The listing builds one solid part. Answer for the finished solid, in the listing's coordinates (mm). Face numbers are marked on the shaded views. A direction names the side the tool comes from. Round coordinates to 2 decimals unless told otherwise and drop trailing zeros. Write each loop counter-clockwise with the first axis right and the second up, starting at its lowest first coordinate (ties: lowest second). Pieces come first, ordered by that corner, then holes.
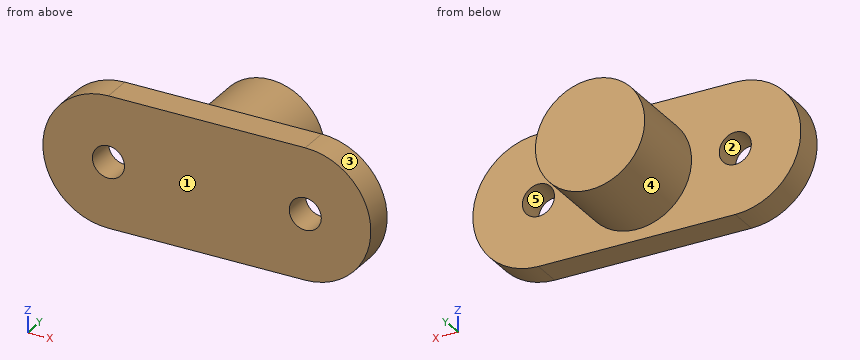
from build123d import *

# Parameters (mm, degrees)
SKETCH1_R           = 1.1
SKETCH1_R_2         = 3.75
BOSS_EXTRUDE3_DEPTH = 2
SKETCH3_R           = 3.75
BOSS_EXTRUDE4_DEPTH = 7.75


with BuildPart() as part:
    # Sketch1 → Boss-Extrude3 (new body)
    with BuildSketch(Plane(origin=(0, 0, 0), x_dir=(1, 0, 0), z_dir=(0, 1, 0))):
        with BuildLine():
            Line((-6.75, 4.499502967), (6.75, 4.499502967))
            ThreePointArc((6.75, 4.499502967), (11.249502967, 0), (6.75, -4.499502967))
            Line((6.75, -4.499502967), (-6.75, -4.499502967))
            ThreePointArc((-6.75, -4.499502967), (-11.249502967, 0), (-6.75, 4.499502967))
        make_face()
        with Locations((-6.75, 0)):
            Circle(SKETCH1_R, mode=Mode.SUBTRACT)
        with Locations((6.75, 0)):
            Circle(SKETCH1_R, mode=Mode.SUBTRACT)
        Circle(SKETCH1_R_2, mode=Mode.SUBTRACT)
    extrude(amount=BOSS_EXTRUDE3_DEPTH)

    # Sketch3 → Boss-Extrude4 (add)
    with BuildSketch(Plane.XZ):
        Circle(SKETCH3_R)
    extrude(amount=-BOSS_EXTRUDE4_DEPTH)


solid = part.part
1. For a pull along X with two mould halves and no side action, classify the marked faces 1, 2 and 3 as released by +X, released by -X, zero draft, split by the parting line, or undercut.
Geometry says:
face 1: zero draft
face 2: undercut
face 3: released by +X
2. Section C-C on x = -7.5 is taken. Determine the outline of the cut face in (y, z).
Geometry says:
outline: (0, -4.44) - (2, -4.44) - (2, -0.8) - (0, -0.8) - close; (0, 0.8) - (2, 0.8) - (2, 4.44) - (0, 4.44) - close
3. Given pin 1 (2.5 mm diameter, centred on x = 6.75, z = 0, fed in from +Y); pin 2 (2 mm diameter, centred on x = 2.5, y = 3.5, fed in from +Z); pin 3 (2 mm diameter, centred on y = 6, z = 2.5, fed in from +X), each flat-ended and moving along its own axis, determine where each tip first touches the part or whether it passes through.
Geometry says:
pin 1: stops at y = 2
pin 2: stops at z = 3.44
pin 3: stops at x = 3.44
4. A tool of negligible diameter and unlimited length cuts with its end or side. For the marked faces 4 and 5, from which of +Z, -Z, +X, -X, +Y, -Y can it reach the whole face along a straight path? Write none if from no direction.
Geometry says:
face 4: +Y
face 5: +Y, -Y
5. Section A-A on z = 0 is taken. Determine the outline of the cut face in (x, y), plus the area to 3 significant figures.
Geometry says:
outline: (-11.25, 0) - (-7.85, 0) - (-7.85, 2) - (-11.25, 2) - close; (-5.65, 0) - (5.65, 0) - (5.65, 2) - (3.75, 2) - (3.75, 7.75) - (-3.75, 7.75) - (-3.75, 2) - (-5.65, 2) - close; (7.85, 0) - (11.25, 0) - (11.25, 2) - (7.85, 2) - close
area: 79.3 mm2
6. Section D-D on z = 1.5 is taken. Determine the outline of the cut face in (x, y).
Geometry says:
outline: (-10.99, 0) - (10.99, 0) - (10.99, 2) - (3.44, 2) - (3.44, 7.75) - (-3.44, 7.75) - (-3.44, 2) - (-10.99, 2) - close
7. Straight lines are drawn through the part: line 1 along X through (y, z) = (0.65, 0); line 2 along Z through (x, y) = (-6.75, 0.6); line 3 along Y through (x, z) = (-8.5, -0.75). For each, find the intervals that lie inside material, in ascending order.
Geometry says:
line 1: x = -11.25 to -7.85, -5.65 to 5.65, 7.85 to 11.25
line 2: z = -4.5 to -1.1, 1.1 to 4.5
line 3: y = 0 to 2
8. Section B-B on x = 0 is taken. Determine the outline of the cut face in (y, z).
Geometry says:
outline: (0, -4.5) - (2, -4.5) - (2, -3.75) - (7.75, -3.75) - (7.75, 3.75) - (2, 3.75) - (2, 4.5) - (0, 4.5) - close
